Here's how the part is built. I have some questions about the finished solid (model axes, mm). Face numbers are marked on the shaded views. A direction names the side the tool comes from. Coordinates: 2 decimals unless noted, no trailing zeros. Use a Markdown table: item, result. Add a question column.
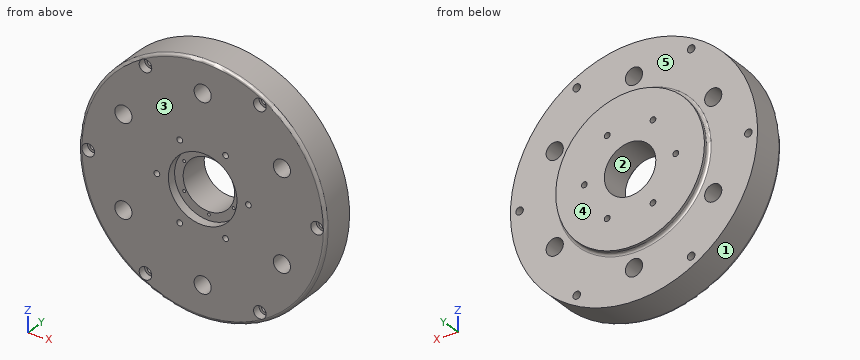
```python
from build123d import *

# Parameters (mm, degrees)
SKETCH_1_R                = 108
SKETCH_1_R_2              = 22.5
EXTRUDE_1_DEPTH           = 30
SKETCH_2_R                = 65
SKETCH_2_R_2              = 22.5
EXTRUDE_2_DEPTH           = 5
SKETCH_6_R                = 30
CUT_EXTRUDE_2_DEPTH       = 8
FILLET_1_R                = 2.5
SKETCH_3_R                = 7.5
CUT_EXTRUDE_1_DEPTH       = 156.653461253
HOLE_WIZARD_M6_1_D        = 5
HOLE_WIZARD_2_D           = 6.6
HOLE_WIZARD_2_CBORE_D     = 11
HOLE_WIZARD_2_CBORE_DEPTH = 7
PATTERN_CIRCULAR_1_COUNT  = 6


with BuildPart() as part:
    # 草图1 → 凸台-拉伸1 (new body)
    with BuildSketch(Plane(origin=(0, 0, 0), x_dir=(1, 0, 0), z_dir=(0, 1, 0))):
        with Locations(Location((0, 0, 0), (0, 0, 270))):
            Circle(SKETCH_1_R)
        with Locations(Location((0, 0, 0), (0, 0, 270))):
            Circle(SKETCH_1_R_2, mode=Mode.SUBTRACT)
    extrude(amount=EXTRUDE_1_DEPTH)

    # 草图2 → 凸台-拉伸2 (add)
    with BuildSketch(Plane(origin=(0, 30, 0), x_dir=(1, 0, 0), z_dir=(0, 1, 0))):
        with Locations(Location((0, 0, 0), (0, 0, 270))):
            Circle(SKETCH_2_R)
        with Locations(Location((0, 0, 0), (0, 0, 270))):
            Circle(SKETCH_2_R_2, mode=Mode.SUBTRACT)
    extrude(amount=EXTRUDE_2_DEPTH)

    # 草图6 → 切除-拉伸2 (cut)
    with BuildSketch(Plane.XZ):
        with Locations(Location((0, 0, 0), (0, 0, 270))):
            Circle(SKETCH_6_R)
    extrude(amount=-CUT_EXTRUDE_2_DEPTH, mode=Mode.SUBTRACT)

    # 圆角1
    fillet_1_edges = [part.edges().sort_by_distance(p)[0] for p in [
        (0, 30, -65),
        (0, 0, -108),
    ]]
    fillet(fillet_1_edges, radius=FILLET_1_R)

    # 草图3 → 切除-拉伸1 (cut, through all)
    with BuildSketch(Plane(origin=(0, 30, 0), x_dir=(1, 0, 0), z_dir=(0, 1, 0))):
        with Locations(Location((0, 80, 0), (0, 0, 270))):
            Circle(SKETCH_3_R)
    cut_extrude_1 = extrude(amount=-CUT_EXTRUDE_1_DEPTH, mode=Mode.SUBTRACT)

    # M6 螺纹孔1 (through all)
    with Locations(Plane(origin=(0, 0, 0), x_dir=(-1, 0, 0), z_dir=(0, -1, 0))):
        with Locations((40, 0)):
            hole_wizard_m6_1 = Hole(HOLE_WIZARD_M6_1_D / 2)

    # 打孔尺寸(%根据)内六角圆柱头螺钉的类型2 (through all)
    with Locations(Plane(origin=(0, 0, 0), x_dir=(-1, 0, 0), z_dir=(0, -1, 0))):
        with Locations((100, 0)):
            hole_wizard_2 = CounterBoreHole(HOLE_WIZARD_2_D / 2, HOLE_WIZARD_2_CBORE_D / 2, HOLE_WIZARD_2_CBORE_DEPTH)

    # 草图11 → M3 螺纹孔1 (revolve, cut)
    with BuildSketch(Plane(origin=(0, 8, -25), x_dir=(0, 0, -1), z_dir=(1, 0, 0))):
        Polygon((0, 0), (0, 8.251075774), (1.25, 7.5), (1.25, 0), align=None)
    hole_wizard_m3_1 = revolve(axis=Axis((0, 1.65, -25), (0, 1, 0)), mode=Mode.SUBTRACT)

    # 阵列(圆周)1: 切除-拉伸1, M6 螺纹孔1, 打孔尺寸(%根据)内六角圆柱头螺钉的类型2, M3 螺纹孔1 ×6 about axis
    pattern_circular_1_axis = Axis((0, 0, 0), (0, 1, 0))
    add([cut_extrude_1.rotate(pattern_circular_1_axis, i * 360 / PATTERN_CIRCULAR_1_COUNT) for i in range(1, PATTERN_CIRCULAR_1_COUNT)], mode=Mode.SUBTRACT)
    add([hole_wizard_m6_1.rotate(pattern_circular_1_axis, i * 360 / PATTERN_CIRCULAR_1_COUNT) for i in range(1, PATTERN_CIRCULAR_1_COUNT)], mode=Mode.SUBTRACT)
    add([hole_wizard_2.rotate(pattern_circular_1_axis, i * 360 / PATTERN_CIRCULAR_1_COUNT) for i in range(1, PATTERN_CIRCULAR_1_COUNT)], mode=Mode.SUBTRACT)
    add([hole_wizard_m3_1.rotate(pattern_circular_1_axis, i * 360 / PATTERN_CIRCULAR_1_COUNT) for i in range(1, PATTERN_CIRCULAR_1_COUNT)], mode=Mode.SUBTRACT)


solid = part.part
```
Q1. Suppose I cut it at A-A, the plane z = 40. State how many separate pieces and enclosed holes the cut face has, and give its area (3 significant figures).
Q2. Please list where these lines run through material, in increasing order: line 1 (Z direction, x = 20, y = 12.5); line 2 (Y direction, x = -67, z = -67); line 3 (Z direction, x = 16, y = 15).
Q3. Will these pins go through, and if not, where does the flat tip stop? pin 1 (3.5 mm diameter, centred on x = 52.5, z = -86.5, fed in from -Y); pin 2 (10 mm diameter, centred on x = -52, y = 23.5, fed in from -Z); pin 3 (6 mm diameter, centred on y = 26.5, z = -55.5, fed in from +X); pin 4 (13.5 mm diameter, centred on x = -69.28, z = -40, fed in from +Y).
Q4. Which directions (+Z, -Z, +X, -X, +Y, -Y) give clear straight access to the entire face, cutting with the end or side of a thin tool? Please do the marked faces 4 and 5.
Q5. Thinking about a two-plate mould opening in X: for the marked faces 1, 2 and 3, which applies, released by +X, released by -X, zero draft, split by the parting line, or undercut?
Answer key:
| question | item | result |
|---|---|---|
| 1 | separate pieces | 3 |
| 1 | enclosed holes | 0 |
| 1 | area | 5,630 mm^2 |
| 2 | line 1 | z = -106.13 to -37.14, -32.14 to -10.31, 10.31 to 32.14, 37.14 to 106.13 |
| 2 | line 2 | y = 0 to 30 |
| 2 | line 3 | z = -106.81 to -15.82, 15.82 to 106.81 |
| 3 | pin 1 | stops at y = 7 |
| 3 | pin 2 | stops at z = -97.24 |
| 3 | pin 3 | stops at x = 94.38 |
| 3 | pin 4 | passes through |
| 4 | face 4 | +Z, -Z, +X, -X, +Y |
| 4 | face 5 | +Y |
| 5 | face 1 | split by the parting line |
| 5 | face 2 | undercut |
| 5 | face 3 | zero draft |
